from build123d import *

# Parameters (mm, degrees)
F0_W     = 129.8851817846
F0_H     = 77.667824924
F0_W_2   = 55.5083644576
F0_H_2   = 7.4596218765
F0_W_3   = 55.5083635263
F1_DEPTH = 50
F0_H_3   = 31.1548877507
F2_DEPTH = 2.5
F4_D     = 5.5
F4_DEPTH = 69.1122023778
F5_D     = 5.5


with BuildPart() as f1:
    # F0 (on Top) → F1 (new body)
    with BuildSketch(Plane.XY):
        Rectangle(F0_W, F0_H)
        Polygon((-59.6769750118, 3.7298109382), (-59.6769750118, 34.884698689), (-4.1686114855, 34.884698689), (4.1686105542, 34.884698689), (59.6769750118, 34.884698689), (59.6769750118, 3.7298109382), (59.6769750118, -3.7298109382), (59.6769750118, -34.884698689), (4.1686105542, -34.884698689), (-4.1686114855, -34.884698689), (-59.6769750118, -34.884698689), (-59.6769750118, -3.7298109382), align=None, mode=Mode.SUBTRACT)
        with Locations((31.922792783, 0)):
            Rectangle(F0_W_2, F0_H_2)
        with Locations((-31.9227932487, 0)):
            Rectangle(F0_W_3, F0_H_2)
        Polygon((4.1686105542, 34.884698689), (-4.1686114855, 34.884698689), (-4.1686114855, 3.7298109382), (-4.1686114855, -3.7298109382), (-4.1686114855, -34.884698689), (4.1686105542, -34.884698689), (4.1686105542, -3.7298109382), (4.1686105542, 3.7298109382), align=None)
    extrude(amount=F1_DEPTH)

    # F0 (on Top) → F2 (join)
    with BuildSketch(Plane.XY):
        Rectangle(F0_W, F0_H)
        Polygon((-59.6769750118, 3.7298109382), (-59.6769750118, 34.884698689), (-4.1686114855, 34.884698689), (4.1686105542, 34.884698689), (59.6769750118, 34.884698689), (59.6769750118, 3.7298109382), (59.6769750118, -3.7298109382), (59.6769750118, -34.884698689), (4.1686105542, -34.884698689), (-4.1686114855, -34.884698689), (-59.6769750118, -34.884698689), (-59.6769750118, -3.7298109382), align=None, mode=Mode.SUBTRACT)
        with Locations((-31.9227932487, -19.3072548136)):
            Rectangle(F0_W_3, F0_H_3)
        with Locations((-31.9227932487, 19.3072548136)):
            Rectangle(F0_W_3, F0_H_3)
        with Locations((31.922792783, -19.3072548136)):
            Rectangle(F0_W_2, F0_H_3)
        with Locations((31.922792783, 19.3072548136)):
            Rectangle(F0_W_2, F0_H_3)
        with Locations((31.922792783, 0)):
            Rectangle(F0_W_2, F0_H_2)
        Polygon((4.1686105542, 34.884698689), (-4.1686114855, 34.884698689), (-4.1686114855, 3.7298109382), (-4.1686114855, -3.7298109382), (-4.1686114855, -34.884698689), (4.1686105542, -34.884698689), (4.1686105542, -3.7298109382), (4.1686105542, 3.7298109382), align=None)
        with Locations((-31.9227932487, 0)):
            Rectangle(F0_W_3, F0_H_2)
    extrude(amount=-F2_DEPTH)

    # F4 (through all, one way)
    with BuildSketch(Plane(origin=(-4.1686114855, 0, 0), x_dir=(0, -1, 0), z_dir=(-1, 0, 0))):
        with Locations((21.7673890293, 25), (-21.2901681662, 25)):
            Circle(F4_D / 2)
    extrude(amount=-F4_DEPTH, mode=Mode.SUBTRACT)

    # F5 (through all)
    with Locations(Plane(origin=(-4.1686114855, 0, 0), x_dir=(0, -1, 0), z_dir=(1, 0, 0))):
        with Locations((-21.2901681662, -25), (21.7673890293, -25)):
            Hole(F5_D / 2)


solid = f1.part
Part model, mm, in its own coordinate system. A direction names the side the tool comes from. Round coordinates to 2 decimals unless told otherwise and drop trailing zeros. Order: outer loops, then holes, each group sorted by start corner. A loop starts at its lowest first (then second) coordinate and runs counter-clockwise, first axis right, second up. Notation, with made-up numbers: (-6, -17.5) -> (37, -17.5) arc R30 ccw to (37, 9.5) -> close; hole circle Ø3 at (-3, 9.5). An arc over 180 degrees is marked (long way). Put each result on its own line as item: value.
Q1. Tool access for faces 4 (the face through (62.273, 24.038, 25.121)), 5 (the face through (32, 3.73, 25)): list every direction of +Z, -Z, +X, -X, +Y, -Y with a clear straight run to the whole face (end or side of a thin tool).
From the geometry:
face 4: +X, -X
face 5: +Z
Q2. Pull direction Y, two halves, no side cores. Call faces 1 (the face through (-64.943, -1, 24)), 2 (the face through (-4.169, -16, 25)), 3 (the face through (-1, -38.834, 24)): pulls with the +Y half, pulls with the -Y half, needs draft (parallel to the pull), parting line crosses it, or undercut.
From the geometry:
face 1: needs draft
face 2: undercut
face 3: pulls with the -Y half
Q3. Band-saw the part on A-A (z = 47). Give the cut face in (x, y).
From the geometry:
outline: (-64.94, -38.83) -> (64.94, -38.83) -> (64.94, 38.83) -> (-64.94, 38.83) -> close; hole (-59.68, -34.88) -> (-4.17, -34.88) -> (-4.17, -3.73) -> (-59.68, -3.73) -> close; hole (-59.68, 3.73) -> (-4.17, 3.73) -> (-4.17, 34.88) -> (-59.68, 34.88) -> close; hole (4.17, -34.88) -> (59.68, -34.88) -> (59.68, -3.73) -> (4.17, -3.73) -> close; hole (4.17, 3.73) -> (59.68, 3.73) -> (59.68, 34.88) -> (4.17, 34.88) -> close
Q4. Wall check: line 1 (X direction, y = -10.5, z = 14.5); line 2 (Y direction, x = 19.5, z = 10); line 3 (Y direction, x = 63.75, z = 25). Give the ranges that are in metal, low to high. Write a range as [from, to].
From the geometry:
line 1: x = [-64.94, -59.68], [-4.17, 4.17], [59.68, 64.94]
line 2: y = [-38.83, -34.88], [-3.73, 3.73], [34.88, 38.83]
line 3: y = [-38.83, -24.52], [-19.02, 18.54], [24.04, 38.83]
Q5. Band-saw the part on D-D (z = 25). State how many separate pieces and enclosed holes the cut face has, and give its area (3 significant figures).
From the geometry:
separate pieces: 3
enclosed holes: 0
area: 2,960 mm2
Q6. Band-saw the part on C-C (x = -12.5). Give the cut face in (y, z), and give its area (3 significant figures).
From the geometry:
outline: (-38.83, -2.5) -> (38.83, -2.5) -> (38.83, 50) -> (34.88, 50) -> (34.88, 0) -> (3.73, 0) -> (3.73, 50) -> (-3.73, 50) -> (-3.73, 0) -> (-34.88, 0) -> (-34.88, 50) -> (-38.83, 50) -> close
area: 962 mm2
Q7. Band-saw the part on B-B (y = -26.5). Give the cut face in (x, z), and give its area (3 significant figures).
From the geometry:
outline: (-64.94, -2.5) -> (64.94, -2.5) -> (64.94, 50) -> (59.68, 50) -> (59.68, 0) -> (4.17, 0) -> (4.17, 50) -> (-4.17, 50) -> (-4.17, 0) -> (-59.68, 0) -> (-59.68, 50) -> (-64.94, 50) -> close
area: 1,270 mm2
Q8. Pin check, flat tip, straight feed: pin 1 Ø1.5 at (x, y) = (5.5, 8.5) entering from +Z. Stop position of the tip, or through.
From the geometry:
pin 1: stops at z = 0
